Part model, mm, in its own coordinate system. A direction names the side the tool comes from. Give positions to 0.01 mm unless a question says otherwise; leave off trailing zeros. Order: outer loops, then holes, each group sorted by start corner. A loop starts at its lowest first (then second) coordinate and runs counter-clockwise, first axis right, second up. Notation, with made-up numbers: M 23.5,-18 L 64.5,-18 A25 ccw 64.5,7 Z; hole C 41.25,-4 d6. An arc over 180 degrees is marked long. Answer as a JSON object with one key per item and string values.
from build123d import *

# Parameters (mm, degrees)
SKETCH2_W           = 647.7
SKETCH2_H           = 342.9
BOSS_EXTRUDE1_DEPTH = 323.85
SHELL1_T            = -19.05


with BuildPart() as part:
    # Sketch2 → Boss-Extrude1 (new body)
    with BuildSketch(Plane(origin=(0, 0, 0), x_dir=(1, 0, 0), z_dir=(0, 1, 0))):
        Rectangle(SKETCH2_W, SKETCH2_H)
    extrude(amount=BOSS_EXTRUDE1_DEPTH)

    # Shell1
    shell1_openings = [part.faces().sort_by_distance(p)[0] for p in [
        (0, 323.85, 0),
    ]]
    offset(amount=SHELL1_T, openings=shell1_openings, kind=Kind.INTERSECTION)


solid = part.part
1. Two-plate mould, pull along Z, no slides. Class faces 3 (the flat face through (-4, 169, -152.4)), 4 (the flat face through (-5, 160, 171.45)), 5 (the flat face through (-323.85, 160, 2)): +Z half, -Z half, draft (parallel to the pull), parting line (faces both ways), or undercut.
Worked answers:
{"face 3": "undercut", "face 4": "+Z half", "face 5": "draft"}
2. Which spindle directions (+Z, -Z, +X, -X, +Y, -Y) get a long thin tool onto all of the face, cutting with end or side? Do faces 1 (the flat face through (-2, 323.85, -153)), 2 (the flat face through (-304.8, 169, 2)). Say none if no direction does.
Worked answers:
{"face 1": "+Z, -Z, +X, -X, +Y", "face 2": "+Y"}
3. Probe line 1 along Z through (x, y) = (46, 190.5); line 2 along X through (y, z) = (25, -141); line 3 along Y through (x, z) = (59.5, -50). List the from-to ranges inside material, lowest first.
Worked answers:
{"line 1": "z = -171.45 to -152.4, 152.4 to 171.45", "line 2": "x = -323.85 to -304.8, 304.8 to 323.85", "line 3": "y = 0 to 19.05"}
4. Cut at A-A on y = 159.5. Give the cut face in (x, z), plus the area to 3 significant figures.
Worked answers:
{"outline": "M -323.85,-171.45 L 323.85,-171.45 L 323.85,171.45 L -323.85,171.45 Z; hole M -304.8,-152.4 L 304.8,-152.4 L 304.8,152.4 L -304.8,152.4 Z", "area": "36,300 mm^2"}
5. Pin check, flat tips, straight feed: P1, Ø1.5, axis at x = -203.5, z = -110, coming from the -Y side; P2, Ø12, axis at x = -109.5, z = 68.5, coming from the +Y side. Stop position of each tip, or through.
Worked answers:
{"P1": "stops at y = 0", "P2": "stops at y = 19.05"}
6. Cut at C-C on z = 127.5. Give the cut face in (x, y).
Worked answers:
{"outline": "M -323.85,0 L 323.85,0 L 323.85,323.85 L 304.8,323.85 L 304.8,19.05 L -304.8,19.05 L -304.8,323.85 L -323.85,323.85 Z"}
7. Cut at B-B on x = 114.5. Give the cut face in (y, z).
Worked answers:
{"outline": "M 0,-171.45 L 323.85,-171.45 L 323.85,-152.4 L 19.05,-152.4 L 19.05,152.4 L 323.85,152.4 L 323.85,171.45 L 0,171.45 Z"}
